Could you check a few things on this drawing? It's one solid part, dimensions in mm from its lowest x, y, z. A direction names the side the tool comes from. Coordinates: 2 decimals unless noted, no trailing zeros. Write each loop counter-clockwise with the first axis right and the second up, starting at its lowest first coordinate (ties: lowest second). Pieces come first, ordered by that corner, then holes. Notation, with made-up numbers: (67, -34) - (117, -34) arc R13 cw to (117, -13) - close; hole circle Ø10 at (13.25, 10). An arc over 180 degrees is marked (long way). Use one line per item in the form item = value. Start each with the question number.
(1) If we section it at C-C on z = 33: Please give me the cut outline in (x, y).
(2) For pin 1 Ø1.5 at (y, z) = (18, 65.5) entering from -X; pin 2 Ø8 at (y, z) = (43, 59) entering from +X; pin 3 Ø3 at (x, z) = (44, 42) entering from +Y; pin 4 Ø6 at (y, z) = (20, 90) entering from +X, each with a flat end and sliding along its axis, tell me the tip position at first contact or that it passes through.
(3) If I drill on probe 1 along Z at (x, y) = (122, 11); probe 2 along X at (y, z) = (15, 83); probe 3 along X at (y, z) = (18.5, 34.5), over which ranges is the centre line in solid material (lowest first)? Write a range as from..to.
(4) On a 3-axis mill with a long thin cutter (end or side, diameter ignored), from which of +Z, -Z, +X, -X, +Y, -Y can I reach the whole of each face in a straight line? I mean the marked faces 5, 6, 7 and 8. Say none if no direction works.
(5) If we section it at A-A on z = 10: Please give me the cut outline in (x, y).
(6) Thinking about a two-plate mould opening in X: for the marked faces 1, 2, 3 and 4, which applies, pulls with the +X half, pulls with the -X half, needs draft (parallel to the pull), parting line crosses it, or undercut?
(7) If we section it at B-B on x = 98: Please give me the cut outline in (y, z).
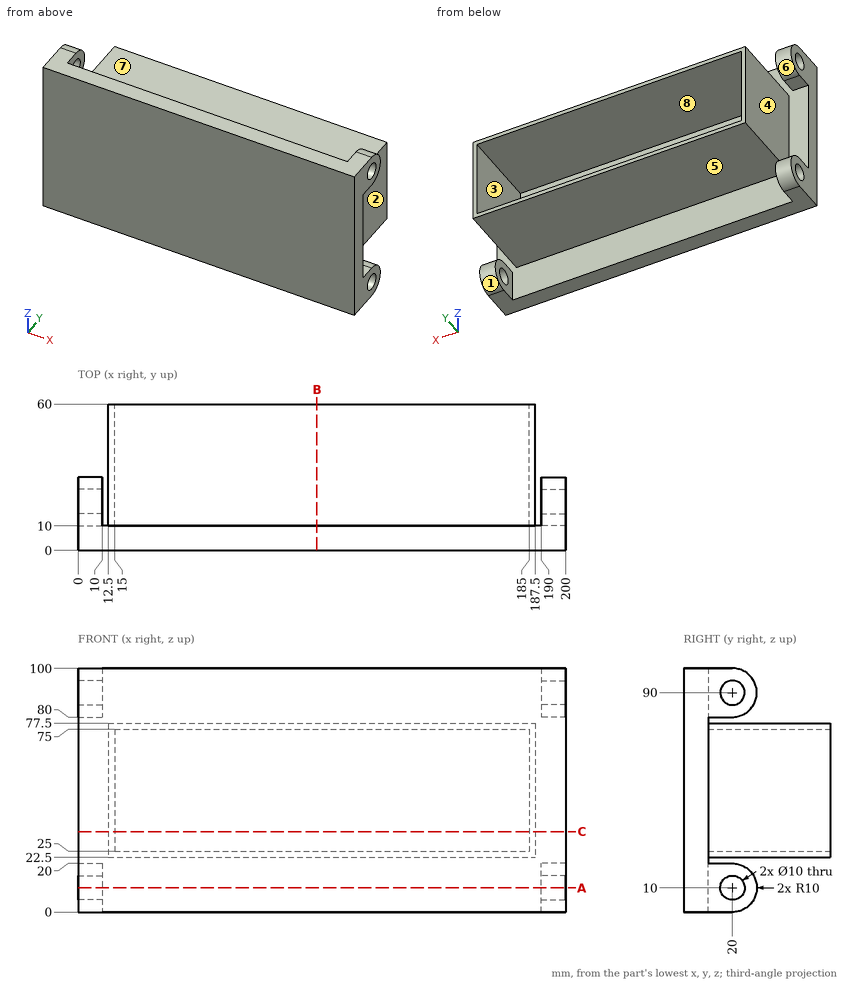
Reported:
q1.outline = (0, 0) - (200, 0) - (200, 10) - (187.5, 10) - (187.5, 60) - (185, 60) - (185, 10) - (15, 10) - (15, 60) - (12.5, 60) - (12.5, 10) - (0, 10) - close
q2.pin_1 = 12.5
q2.pin_2 = 187.5
q2.pin_3 = 10
q2.pin_4 = through
q3.probe_1 = 22.5..25, 75..77.5
q3.probe_2 = 0..10, 190..200
q3.probe_3 = 12.5..15, 185..187.5
q4.face_5 = -Z, +X, -X, +Y
q4.face_6 = +X, -X, +Y
q4.face_7 = +Z, +X, -X, +Y
q4.face_8 = +Y
q5.outline = (0, 0) - (200, 0) - (200, 15) - (190, 15) - (190, 10) - (10, 10) - (10, 15) - (0, 15) - close; (0, 25) - (10, 25) - (10, 30) - (0, 30) - close; (190, 25) - (200, 25) - (200, 30) - (190, 30) - close
q6.face_1 = needs draft
q6.face_2 = pulls with the +X half
q6.face_3 = undercut
q6.face_4 = pulls with the -X half
q7.outline = (0, 0) - (10, 0) - (10, 22.5) - (60, 22.5) - (60, 25) - (10, 25) - (10, 75) - (60, 75) - (60, 77.5) - (10, 77.5) - (10, 100) - (0, 100) - close
